Geometry: final body of the model. Coordinates: model frame, mm. Face numbers are marked on the shaded views. A direction names the side the tool comes from. Give positions to 0.01 mm unless a question says otherwise; leave off trailing zeros. Write each loop counter-clockwise with the first axis right and the second up, starting at its lowest first coordinate (ties: lowest second). Pieces come first, ordered by that corner, then holes. Notation, with made-up numbers: M 31,14.5 L 66,14.5 A30 cw 66,53.5 Z; hole C 66,-27.5 d10. An arc over 180 degrees is marked long. Use a Markdown table: item, result. Add a question column.
1) Set-up query: the marked faces 4 and 5. Return all of +Z, -Z, +X, -X, +Y, -Y with unobstructed straight access to the full face (end or side cutting, diameter ignored); none if empty.
2) Section A-A on z = 31. Return the cut outline in (x, y), then the cut area to 3 significant figures.
3) Draft query along X for the marked faces 1, 2 and 3. Return one class per face: +X half, -X half, draft (parallel to the pull), parting line (faces both ways), or undercut.
4) Section B-B on x = -18. Return the cut outline in (y, z), then the cut area to 3 significant figures.
5) Pin query (flat end, axial travel): pin 1 (10 mm diameter, centred on x = -25.5, z = 12.5, fed in from -Y); pin 2 (1.7 mm diameter, centred on x = -25.29, z = 18.77, fed in from +Y); pin 3 (4 mm diameter, centred on x = -11.5, z = 11.5, fed in from +Y); pin 4 (3.5 mm diameter, centred on x = -10.5, z = 31, fed in from -Y). Return the tip coordinate at first contact, or that it passes through.
6) Section C-C on y = -7.5. Return the cut outline in (x, z).
7) Line query: line 1 (Z direction, x = -10, y = 13); line 2 (Z direction, x = -10, y = 10.25); line 3 (X direction, y = 12.5, z = 31). Output: solid intervals per line, ascending.
8) Section D-D on x = -10. Return the cut outline in (y, z).
```python
from build123d import *

# Parameters (mm, degrees)
SKETCH024_R             = 3.5
SKETCH024_R_2           = 1.9
PAD012_DEPTH            = 12
SKETCH025_R             = 2
SKETCH025_R_2           = 0.972006
PAD013_DEPTH            = 3
PAD014_DEPTH            = 22
PAD015_DEPTH            = 0.5
BODY006_PLACEMENT_ANGLE = 22.5


with BuildPart() as part:
    # Sketch024 → Pad012 (new body)
    with BuildSketch(Plane.XZ.offset(-7)):
        Circle(SKETCH024_R)
        Circle(SKETCH024_R_2, mode=Mode.SUBTRACT)
    extrude(amount=PAD012_DEPTH)

    # Sketch025 → Pad013 (join)
    with BuildSketch(Plane.XZ.offset(-1)):
        with BuildLine():
            Line((3.591196, 0.770117), (3.591196, -0.770117))
            ThreePointArc((1.361313, -3), (2.938078, -2.346882), (3.591196, -0.770117))
            Line((-12.451851, -3), (1.361313, -3))
            ThreePointArc((-12.451851, -3), (-13.518451, -3.22331), (-14.40589, -3.855731))
            Line((-14.40589, -3.855731), (-15.625704, -5.177633))
            ThreePointArc((-15.625704, -5.177633), (-15.890477, -5.83085), (-15.658609, -6.496457))
            Line((-15.658609, -6.496457), (-4.807646, -19.501059))
            Line((-4.807646, -19.501059), (-11.027147, -18.20942))
            Line((-19.99501, -7.462236), (-11.027147, -18.20942))
            ThreePointArc((-19.821704, -3.713124), (-20.637136, -5.553991), (-19.99501, -7.462236))
            Line((-14.397367, 1.685472), (-19.821704, -3.713124))
            ThreePointArc((-11.21311, 3), (-12.93557, 2.658446), (-14.397367, 1.685472))
            Line((-11.21311, 3), (-4.42391, 3))
            Line((-4.42391, 3), (1.361313, 3))
            ThreePointArc((3.591196, 0.770117), (2.938078, 2.346882), (1.361313, 3))
        make_face()
        Circle(SKETCH025_R, mode=Mode.SUBTRACT)
        with Locations((-18.806547, -5.445875)):
            Circle(SKETCH025_R_2, mode=Mode.SUBTRACT)
    extrude(amount=PAD013_DEPTH)

    # Sketch026 → Pad014 (join)
    with BuildSketch(Plane.XZ):
        with BuildLine():
            ThreePointArc((-12.313913, -15.505081), (-5.478083, -19.027102), (2.184032, -19.679177))
            ThreePointArc((2.426703, -21.865752), (3.398655, -20.651129), (2.184032, -19.679177))
            ThreePointArc((-13.682126, -17.227868), (-6.086758, -21.141224), (2.426703, -21.865752))
            ThreePointArc((-12.313913, -15.505081), (-13.859413, -15.682368), (-13.682126, -17.227868))
        make_face()
    extrude(amount=PAD014_DEPTH)

    # Sketch027 → Pad015 (join, symmetric)
    with BuildSketch(Plane.XZ.offset(2)):
        Polygon((-28.80796, -19.352043), (-23.182241, -21.180655), (-12.468725, -18.606313), (-11.456409, -18.159056), (-11.456409, -15.568812), (-22.449142, -14.305279), align=None)
    extrude(amount=PAD015_DEPTH, both=True)


with BuildPart() as part_1:
    # Body006 placement: moved
    add(part.part.moved(Location((-10, 10, 31))).rotate(Axis((-10, 10, 31), (0, -1, 0)), BODY006_PLACEMENT_ANGLE))


solid = part_1.part
```
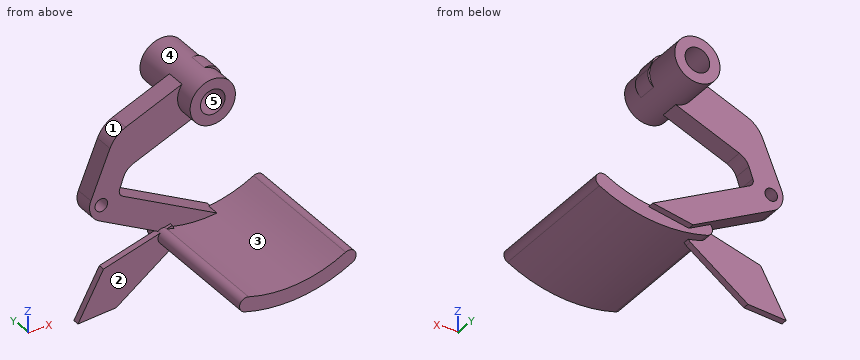
Found:
| question | item | result |
|---|---|---|
| 1 | face 4 | none |
| 1 | face 5 | +Y, -Y |
| 2 | outline | M -17.84,8 L -13.5,8 L -13.5,5 L -11.9,5 L -11.9,17 L -13.5,17 L -13.5,11 L -17.84,11 Z; M -8.1,5 L -6.5,5 L -6.5,8 L -6.23,8 L -6.23,11 L -6.5,11 L -6.5,17 L -8.1,17 Z |
| 2 | area | 52.2 mm² |
| 3 | face 1 | -X half |
| 3 | face 2 | draft |
| 3 | face 3 | undercut |
| 4 | outline | M 7.5,6.42 L 8.5,6.42 L 8.5,11.27 L 7.5,11.27 Z; M 8,12.46 L 11,12.46 L 11,16.92 L 8,16.92 Z; M 8,24.44 L 11,24.44 L 11,30.93 L 8,30.93 Z |
| 4 | area | 37.7 mm² |
| 5 | pin 1 | y = 7.5 |
| 5 | pin 2 | through |
| 5 | pin 3 | y = 11 |
| 5 | pin 4 | y = 5 |
| 6 | outline | M -16.05,9.85 A22 ccw 0.61,11.73 A1.1 ccw -0.45,13.65 A19.8 cw -15.44,11.96 A1.1 ccw Z |
| 7 | line 1 | 27.5 to 29.1, 32.9 to 34.5 |
| 7 | line 2 | 10.57 to 12.73, 27.5 to 29.1, 32.9 to 34.5 |
| 7 | line 3 | -13.5 to -11.9, -8.1 to -6.5 |
| 8 | outline | M -12,9 L 10,9 L 10,10.57 L 11,10.57 L 11,12.73 L 8,12.73 L 8,11.2 L -12,11.2 Z; M 5,27.5 L 17,27.5 L 17,29.1 L 5,29.1 Z; M 5,32.9 L 17,32.9 L 17,34.5 L 5,34.5 Z |
